from build123d import *

# Parameters (mm, degrees)
SCHIZZO1_W                   = 60
SCHIZZO1_H                   = 31
ESTRUSIONE_ESTRUSIONE1_DEPTH = 18
SCHIZZO2_W                   = 13
SCHIZZO2_H                   = 13
ESTRUSIONE_ESTRUSIONE2_DEPTH = 20
SCHIZZO3_W                   = 3
SCHIZZO3_H                   = 3
TAGLIO_ESTRUSIONE1_DEPTH     = 5


with BuildPart() as part:
    # Schizzo1 → Estrusione-Estrusione1 (new body)
    with BuildSketch(Plane(origin=(0, 0, 0), x_dir=(1, 0, 0), z_dir=(0, 1, 0))):
        with Locations((-10.807034353, -6.614779908)):
            Rectangle(SCHIZZO1_W, SCHIZZO1_H)
    extrude(amount=ESTRUSIONE_ESTRUSIONE1_DEPTH)

    # Schizzo2 → Estrusione-Estrusione2 (add)
    with BuildSketch(Plane(origin=(0, 18, 0), x_dir=(1, 0, 0), z_dir=(0, 1, 0))):
        with Locations((-20.307034353, -1.614779908)):
            Rectangle(SCHIZZO2_W, SCHIZZO2_H)
        with Locations((-4.307034353, -1.614779908)):
            Rectangle(SCHIZZO2_W, SCHIZZO2_H)
    extrude(amount=ESTRUSIONE_ESTRUSIONE2_DEPTH)

    # Schizzo3 → Taglio-Estrusione1 (cut)
    with BuildSketch(Plane.ZY.offset(40.807034353)):
        with Locations((-2.885220092, 7.5)):
            Rectangle(SCHIZZO3_W, SCHIZZO3_H)
        with Locations((2.614779908, 7.5)):
            Rectangle(SCHIZZO3_W, SCHIZZO3_H)
        with Locations((10.614779908, 7.5)):
            Rectangle(SCHIZZO3_W, SCHIZZO3_H)
        with Locations((16.114779908, 7.5)):
            Rectangle(SCHIZZO3_W, SCHIZZO3_H)
    extrude(amount=-TAGLIO_ESTRUSIONE1_DEPTH, mode=Mode.SUBTRACT)


solid = part.part
Input: part model. Units: mm. Frame: model coordinates. A direction names the side the tool comes from. Give positions to 0.01 mm unless a question says otherwise; leave off trailing zeros. Loops run counter-clockwise (first coordinate to the right, second up) from the corner with the lowest first, then second, coordinate; pieces in that order, holes last. Notation, with made-up numbers: (-12.5, 26) - (19.5, 26) arc R19 ccw to (19.5, 51) - close; hole circle Ø2 at (61.25, 57). An arc over 180 degrees is marked (long way). Use CSV: the item, a comma, the result in double quotes. Start each with the question number.
Item 1: Section B-B on x = -3. Return loops of the section in (y, z).
Item 2: Reachability of faces 1 (the flat face through (-35.807, 8, 11)), 2 (the flat face through (-10.807, 28, 2)), 3 (the flat face through (-20, 28, 8.115)) from +Z, -Z, +X, -X, +Y, -Y: full face, straight path, thin tool, end or side. Return the list, or none.
Item 3: Section D-D on z = 18.5. Return loops of the section in (x, y).
Item 4: Section A-A on y = 31.5. Return loops of the section in (x, z).
Item 5: Mould query, pull axis X, two halves, no side actions, for faces 4 (the flat face through (-13.807, 28, 2)), 5 (the flat face through (-20, 28, -4.885)), 6 (the flat face through (2.193, 28, 2)), 7 (the flat face through (-35.807, 8, 3)). Classes: pulls with the +X half, pulls with the -X half, needs draft (parallel to the pull), parting line crosses it, or undercut.
Item 6: Line query: line 1 (X direction, y = 34.5, z = 1.5); line 2 (Y direction, x = -37, z = 3.5); line 3 (Y direction, x = 9, z = 11). Output: solid intervals per line, ascending.
Item 7: Section C-C on z = -2.5. Return loops of the section in (x, y).
Item 8: Contact query for flat-ended pins moving along their axis: P1, Ø1.5, axis at x = -37.5, z = 16.5, coming from the +Y side; P2, Ø10.5, axis at y = 26.5, z = 3.5, coming from the -X side; P3, Ø10.5, axis at x = -23, y = 23.5, coming from the -Z side. Output: stop coordinate, or through.
Ans:
1,outline,"(0, -8.89) - (18, -8.89) - (18, -4.89) - (38, -4.89) - (38, 8.11) - (18, 8.11) - (18, 22.11) - (0, 22.11) - close"
2,face 1,"-X"
2,face 2,"+Z, -Z, +Y"
2,face 3,"+Z, +X, -X, +Y"
3,outline,"(-40.81, 0) - (19.19, 0) - (19.19, 18) - (-40.81, 18) - close"
4,outline,"(-26.81, -4.89) - (-13.81, -4.89) - (-13.81, 8.11) - (-26.81, 8.11) - close; (-10.81, -4.89) - (2.19, -4.89) - (2.19, 8.11) - (-10.81, 8.11) - close"
5,face 4,"undercut"
5,face 5,"needs draft"
5,face 6,"pulls with the +X half"
5,face 7,"pulls with the -X half"
6,line 1,"x = -26.81 to -13.81, -10.81 to 2.19"
6,line 2,"y = 0 to 6, 9 to 18"
6,line 3,"y = 0 to 18"
7,outline,"(-40.81, 0) - (19.19, 0) - (19.19, 18) - (2.19, 18) - (2.19, 38) - (-10.81, 38) - (-10.81, 18) - (-13.81, 18) - (-13.81, 38) - (-26.81, 38) - (-26.81, 18) - (-40.81, 18) - (-40.81, 9) - (-35.81, 9) - (-35.81, 6) - (-40.81, 6) - close"
8,P1,"stops at y = 18"
8,P2,"stops at x = -26.81"
8,P3,"stops at z = -4.89"
